Source: CAD feature listing. Evaluate the final solid. Frame: model axes, mm. A direction names the side the tool comes from. Round coordinates to 2 decimals unless told otherwise and drop trailing zeros. Write each loop counter-clockwise with the first axis right and the second up, starting at its lowest first coordinate (ties: lowest second). Pieces come first, ordered by that corner, then holes. Notation, with made-up numbers: (30, -11.75) -> (44, -11.75) arc R34 ccw to (44, 20.25) -> close; hole circle Ø9 at (12, -19.75). An arc over 180 degrees is marked (long way). Put each result on its own line as item: value.
```python
from build123d import *


with BuildPart() as part:
    # Sketch1 → BaseBody (revolve)
    with BuildSketch(Plane.XY):
        with BuildLine():
            Line((0, 3.9624), (0, 7.4676))
            ThreePointArc((0, 7.4676), (0.23062412, 8.02437588), (0.7874, 8.255))
            Line((0.7874, 8.255), (3.9624, 8.255))
            Line((3.9624, 8.255), (3.9624, 6.6675))
            ThreePointArc((3.9624, 6.6675), (3.737893597, 6.125493597), (4.2799, 6.35))
            Line((4.2799, 6.35), (22.6949, 6.35))
            Line((22.6949, 6.35), (23.0124, 6.0325))
            Line((23.0124, 6.0325), (23.0124, 3.175))
            Line((23.0124, 3.175), (0.7874, 3.175))
            ThreePointArc((0.7874, 3.175), (0.23062412, 3.40562412), (0, 3.9624))
        make_face()
    revolve(axis=Axis((0, 0, 0), (1, 0, 0)))


solid = part.part
```
Q1. Draft query along Y for faces 3 (the cylindrical face through (2.397, 7.874, 2.48)), 4 (the cylindrical face through (11.74, -0.69, -3.1)), 5 (the flat face through (0, -3, -3)). Return one class per face: +Y half, -Y half, draft (parallel to the pull), parting line (faces both ways), or undercut.
Ans:
face 3: parting line
face 4: undercut
face 5: draft
Q2. Cut plane C-C on x = 3. Output: boundary loops of the cut face in (y, z) (3 decimals).
Ans:
outline: circle Ø16.51 at (0, 0); hole circle Ø6.35 at (0, 0)
Q3. Material intervals for line 1 (Z direction, x = 9.5, y = 0) (3 decimals); line 2 (Z direction, x = 4.5, y = 5.5); line 3 (Z direction, x = 1, y = -1.5), sorted ascending. Write a range as [from, to].
Ans:
line 1: z = [-6.35, -3.175], [3.175, 6.35]
line 2: z = [-3.17, 3.17]
line 3: z = [-8.12, -2.8], [2.8, 8.12]
Q4. Pin query (flat end, axial travel): pin 1 (4 mm diameter, centred on x = 12, z = 3.5, fed in from +Y); pin 2 (8 mm diameter, centred on x = 11, z = 1, fed in from +Y); pin 3 (2 mm diameter, centred on x = 13.5, y = 1.5, fed in from +Z). Return the tip coordinate at first contact, or that it passes through.
Ans:
pin 1: stops at y = 6.17
pin 2: stops at y = 6.35
pin 3: stops at z = 6.33
Q5. Cut plane D-D on x = 17. Output: boundary loops of the cut face in (y, z) (3 decimals), and give its area (3 significant figures).
Ans:
outline: circle Ø12.7 at (0, 0); hole circle Ø6.35 at (0, 0)
area: 95.0 mm^2
Q6. Reachability of faces 1 (the flat face through (23.012, 3, -3)), 2 (the cylindrical face through (13.62, -1.38, -6.2)) from +Z, -Z, +X, -X, +Y, -Y: full face, straight path, thin tool, end or side. Return the list, or none.
Ans:
face 1: +Z, -Z, +X, +Y, -Y
face 2: +X
